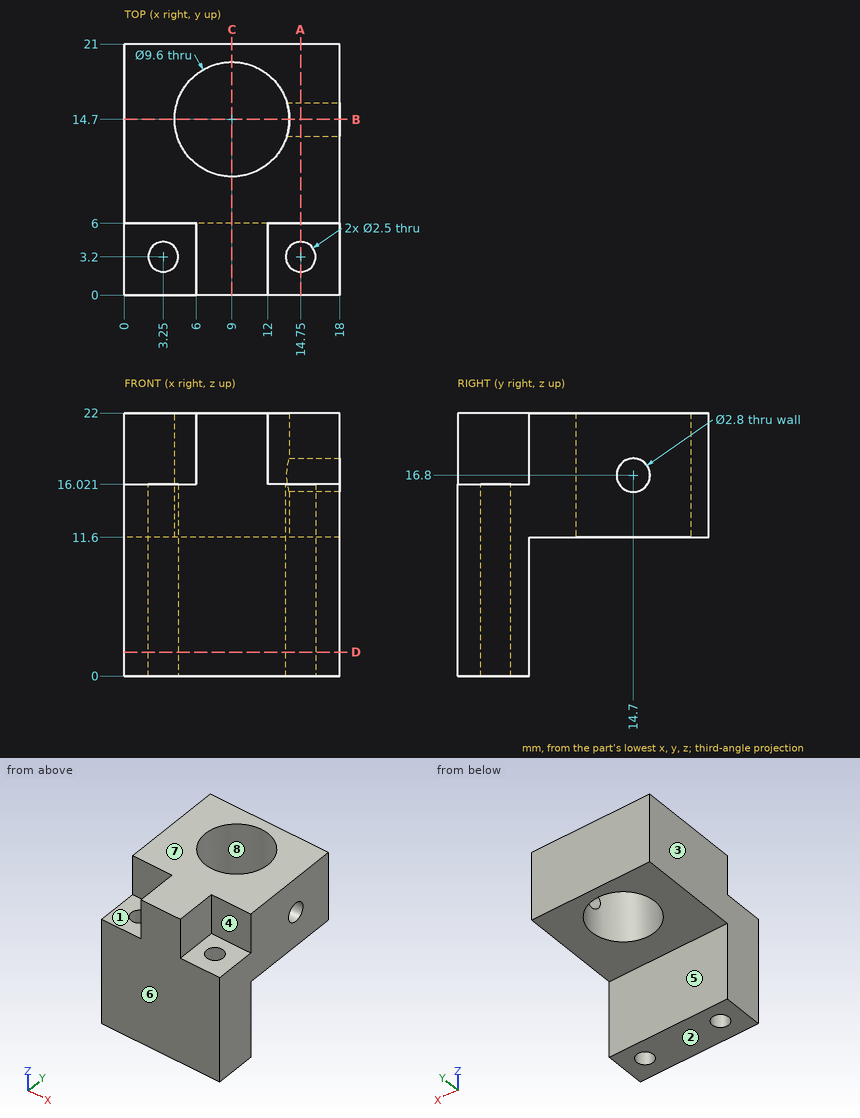
Input: dimensioned drawing with shaded views. Units: mm. Origin: part minimum x, y, z. A direction names the side the tool comes from. Coordinates: 2 decimals unless noted, no trailing zeros. Write each loop counter-clockwise with the first axis right and the second up, starting at its lowest first coordinate (ties: lowest second). Pieces come first, ordered by that corner, then holes. Notation, with made-up numbers: (-37.75, 78.25) -> (12.25, 78.25) arc R12 ccw to (12.25, 97.25) -> close; hole circle Ø8 at (37, 48.5). An arc over 180 degrees is marked (long way). Return JSON: item names as keys, results as strings. Group by question number.
1) Section query A-A, the plane x = 14.75. Return loops of the section in (y, z).
2) Section query B-B, the plane y = 14.7. Return loops of the section in (x, z).
3) Set-up query: the marked faces 1, 2, 3, 4 and 5. Return all of +Z, -Z, +X, -X, +Y, -Y with unobstructed straight access to the full face (end or side cutting, diameter ignored); none if empty.
4) Section query D-D, the plane z = 2. Return loops of the section in (x, y).
5) Contact query for flat-ended pins moving along their axis: P1, Ø3, axis at x = 3.5, y = 1.5, coming from the +Z side; P2, Ø6.5, axis at x = 2, z = 18.5, coming from the -Y side; P3, Ø5, axis at y = 3, z = 19.5, coming from the +X side; P4, Ø1.5, axis at x = 14.75, y = 3.2, coming from the -Z side. Output: stop coordinate, or through.
6) Mould query, pull axis Y, two halves, no side actions, for the marked faces 6, 7 and 8. Classes: +Y half, -Y half, draft (parallel to the pull), parting line (faces both ways), or undercut.
7) Ray query, line 1 along Z through (x, y) = (16.25, 14.7); line 2 along Y through (x, z) = (9, 15.75); line 3 along Y through (x, z) = (14.75, 9.25). Return the intervals inside material, ascending.
8) Section query C-C, the plane x = 9. Return loops of the section in (y, z).
From the geometry:
{
 "1": {"outline": "(0, 0) -> (1.95, 0) -> (1.95, 16.02) -> (0, 16.02) -> close; (4.45, 0) -> (6, 0) -> (6, 11.6) -> (21, 11.6) -> (21, 22) -> (6, 22) -> (6, 16.02) -> (4.45, 16.02) -> close; hole circle Ø2.8 at (14.7, 16.8)"},
 "2": {"outline": "(0, 11.6) -> (4.2, 11.6) -> (4.2, 22) -> (0, 22) -> close; (13.8, 11.6) -> (18, 11.6) -> (18, 15.4) -> (13.8, 15.4) -> close; (13.8, 18.2) -> (18, 18.2) -> (18, 22) -> (13.8, 22) -> close"},
 "3": {"face 1": "+Z, -X, -Y", "face 2": "-Z, +X, -X, +Y, -Y", "face 3": "+Z, -Z, -X, +Y, -Y", "face 4": "+Z, +X, -Y", "face 5": "-Z, +X, -X, +Y"},
 "4": {"outline": "(0, 0) -> (18, 0) -> (18, 6) -> (0, 6) -> close; hole circle Ø2.5 at (3.25, 3.2); hole circle Ø2.5 at (14.75, 3.2)"},
 "5": {"P1": "z = 16.02", "P2": "y = 0", "P3": "x = 12", "P4": "through"},
 "6": {"face 6": "-Y half", "face 7": "draft", "face 8": "undercut"},
 "7": {"line 1": "11.6 to 15.4, 18.2 to 22", "line 2": "0 to 9.9, 19.5 to 21", "line 3": "0 to 1.95, 4.45 to 6"},
 "8": {"outline": "(0, 0) -> (6, 0) -> (6, 11.6) -> (9.9, 11.6) -> (9.9, 22) -> (0, 22) -> close; (19.5, 11.6) -> (21, 11.6) -> (21, 22) -> (19.5, 22) -> close"}
}
